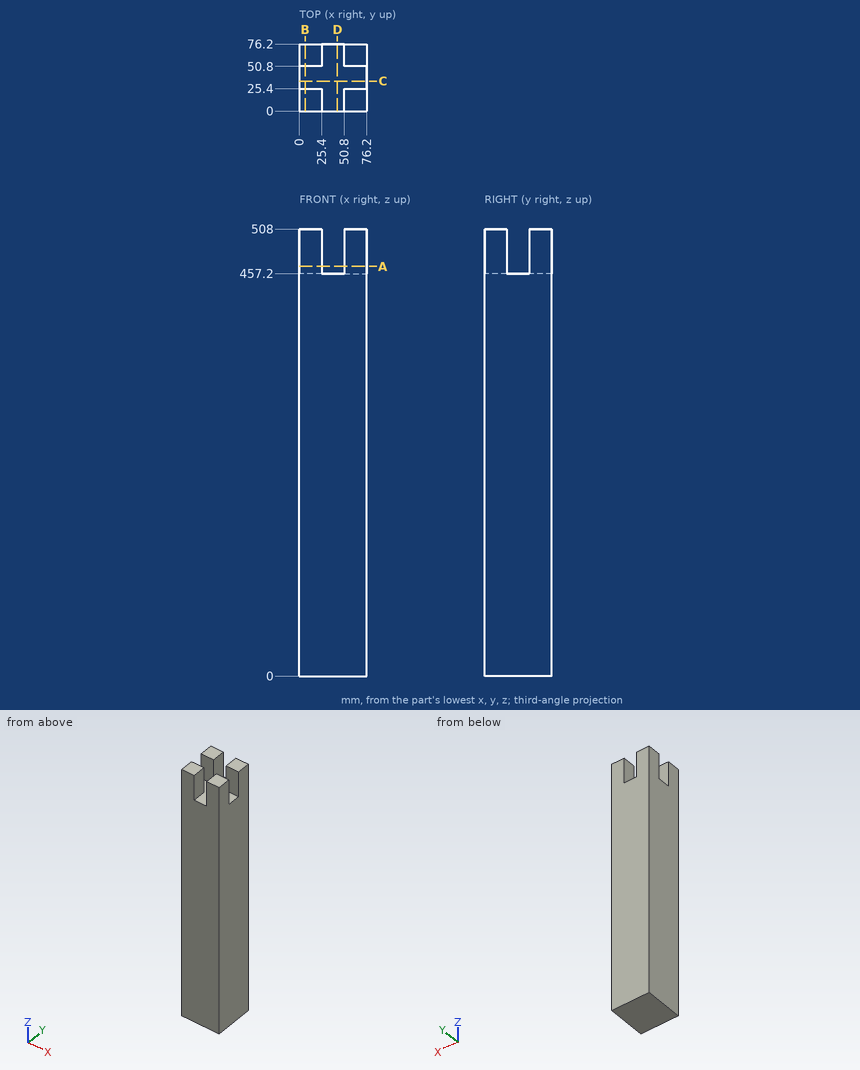
Can you work these out from the drawing? Everything is in mm from the part's minimum corner. Coordinates: 2 decimals unless noted, no trailing zeros. Loops run counter-clockwise (first coordinate to the right, second up) from the corner with the lowest first, then second, coordinate; pieces in that order, holes last.
1) Imagine slicing it at A-A on z = 465.5. List the corners of the cut face in (x, y) for me.
2) For pin 1 (6 mm diameter, centred on x = 41, y = 50, fed in from +Z), with a flat end and sliding along its axis, tell me the tip position at first contact or that it passes through.
3) Imagine slicing it at C-C on y = 34. List the corners of the cut face in (x, z) for me.
4) I need wall thicknesses on probe 1 along Z at (x, y) = (32, 59). Which ranges of the line are inside material? Lowest first, please.
5) Imagine slicing it at B-B on x = 6.5. List the corners of the cut face in (y, z) for me.
Completed:
1. outline: (0, 0) - (25.4, 0) - (25.4, 25.4) - (0, 25.4) - close; (0, 50.8) - (25.4, 50.8) - (25.4, 76.2) - (0, 76.2) - close; (50.8, 0) - (76.2, 0) - (76.2, 25.4) - (50.8, 25.4) - close; (50.8, 50.8) - (76.2, 50.8) - (76.2, 76.2) - (50.8, 76.2) - close
2. pin 1: stops at z = 457.2
3. outline: (0, 0) - (76.2, 0) - (76.2, 457.2) - (0, 457.2) - close
4. probe 1: z = 0 to 457.2
5. outline: (0, 0) - (76.2, 0) - (76.2, 508) - (50.8, 508) - (50.8, 457.2) - (25.4, 457.2) - (25.4, 508) - (0, 508) - close
